```python
from build123d import *

# Parameters (mm, degrees)
POCKET_DEPTH = 12.001


with BuildPart() as part:
    # Sketch → Revolution (revolve)
    with BuildSketch(Plane.XZ):
        Polygon((0, 0), (38, 0), (36, 17), (28, 17), (28, 14), (32, 14), (32, 5), (0, 5), align=None)
    revolve(axis=Axis((0, 0, 0), (0, 0, 1)))

    # Sketch001 (on Face7 of Revolution) → Pocket (cut, through all)
    with BuildSketch(Plane(origin=(0, 0, 5), x_dir=(-1, 0, 0), z_dir=(0, 0, 1))):
        with BuildLine():
            ThreePointArc((28.266588, -15), (32, 0), (28.266588, 15))
            Line((28.266588, 15), (-28.266588, 15))
            ThreePointArc((-28.266588, 15), (-32, 0), (-28.266588, -15))
            Line((28.266588, -15), (-28.266588, -15))
        make_face()
    extrude(amount=POCKET_DEPTH, mode=Mode.SUBTRACT)


solid = part.part
```
Design review of the part built by this model. Coordinates are the model's own, in mm. A direction names the side the tool comes from. Coordinates: 2 decimals unless noted, no trailing zeros. Loops run counter-clockwise (first coordinate to the right, second up) from the corner with the lowest first, then second, coordinate; pieces in that order, holes last.
Q1. Tool access review of faces 4 (the face through (-26, 15, 15)), 5 (the face through (0.1, -28.5, 14)), 6 (the face through (1, 1, 0)): name each direction out of +Z, -Z, +X, -X, +Y, -Y from which nothing blocks a thin tool from reaching the whole face with its end or side.
Reported:
face 4: +Z
face 5: none
face 6: -Z, +X, -X, +Y, -Y
Q2. For pin 1 (1.5 mm diameter, centred on x = -26.5, z = 15, fed in from -Y); pin 2 (2 mm diameter, centred on x = -26.5, z = 12.5, fed in from +Y); pin 3 (1.5 mm diameter, centred on x = -3.5, z = 7.5, fed in from +Y), all flat-tipped, find the tip position at first contact; note any pin that passes through.
Reported:
pin 1: stops at y = -25.5
pin 2: stops at y = 26.17
pin 3: stops at y = 37.06
Q3. To check wall thickness, follow line 1 (Z direction, x = -3, y = -28.5); line 2 (Z direction, x = 1, y = -24.5); line 3 (X direction, y = -16.5, z = 8.75). State the ranges of each line that lie inside material, in increasing order.
Reported:
line 1: z = 0 to 5, 14 to 17
line 2: z = 0 to 5
line 3: x = -33.08 to -27.42, 27.42 to 33.08
Q4. We need section C-C on z = 12. State the section outline as (x, y) points, and give its area (3 significant figures).
Reported:
outline: circle Ø73.18 at (0, 0); hole circle Ø64 at (0, 0)
area: 989 mm2
Q5. We need section D-D on z = 3.25. State the section outline as (x, y) points.
Reported:
outline: circle Ø75.24 at (0, 0)
Q6. We need section B-B on x = 0. State the section outline as (y, z) points, and give its area (3 significant figures).
Reported:
outline: (-38, 0) - (38, 0) - (36, 17) - (28, 17) - (28, 14) - (32, 14) - (32, 5) - (-32, 5) - (-32, 14) - (-28, 14) - (-28, 17) - (-36, 17) - close
area: 514 mm2
Q7. We need section A-A on y = 0. State the section outline as (x, z) points, and give its area (3 significant figures).
Reported:
outline: (-38, 0) - (38, 0) - (36, 17) - (32, 17) - (32, 5) - (-32, 5) - (-32, 17) - (-36, 17) - close
area: 490 mm2
Q8. The part is to be moulded in two halves that separate along Y. For faces 1 (the face through (-22, 19, 17)), 2 (the face through (0, 28, 15)), 3 (the face through (-7.921, -35.673, 12.397)), say which applies: +Y half, -Y half, draft (parallel to the pull), parting line (faces both ways), or undercut.
Reported:
face 1: draft
face 2: undercut
face 3: parting line
